```python
from build123d import *

# Parameters (mm, degrees)
SKETCH1_R           = 15
BOSS_EXTRUDE1_DEPTH = 40
BOSS_EXTRUDE2_START = 20
SKETCH2_R           = 20
BOSS_EXTRUDE2_DEPTH = 30
SKETCH3_R           = 15
BOSS_EXTRUDE3_DEPTH = 40


with BuildPart() as part:
    # Sketch1 → Boss-Extrude1 (new body)
    with BuildSketch(Plane(origin=(0, 0, 0), x_dir=(1, 0, 0), z_dir=(0, 1, 0))):
        with BuildLine():
            Line((-20, -20), (20, -20))
            Line((20, -20), (20, 0))
            ThreePointArc((20, 0), (0, 20), (-20, 0))
            Line((-20, 0), (-20, -20))
        make_face()
        with Locations(Location((0, 0, 0), (0, 0, 270))):
            Circle(SKETCH1_R, mode=Mode.SUBTRACT)
    extrude(amount=BOSS_EXTRUDE1_DEPTH)

    # Sketch2 → Boss-Extrude2 (add)
    with BuildSketch(Plane.XY.offset(BOSS_EXTRUDE2_START)):
        with Locations((0, 20)):
            Circle(SKETCH2_R)
    extrude(amount=BOSS_EXTRUDE2_DEPTH)

    # Sketch3 → Boss-Extrude3 (add)
    with BuildSketch(Plane.ZY.offset(20)):
        with BuildLine():
            Line((50, 40.055924185), (50, 0.055924185))
            Line((50, 0.055924185), (70, 0.055924185))
            ThreePointArc((70, 0.055924185), (90, 20.055924185), (70, 40.055924185))
            Line((70, 40.055924185), (50, 40.055924185))
        make_face()
        with Locations(Location((70, 20.055924185, 0), (0, 0, 270))):
            Circle(SKETCH3_R, mode=Mode.SUBTRACT)
    extrude(amount=-BOSS_EXTRUDE3_DEPTH)


solid = part.part
```
The listing builds one solid part. Answer for the finished solid, in the listing's coordinates (mm). A direction names the side the tool comes from. Round coordinates to 2 decimals unless told otherwise and drop trailing zeros. Order: outer loops, then holes, each group sorted by start corner. A loop starts at its lowest first (then second) coordinate and runs counter-clockwise, first axis right, second up. Notation, with made-up numbers: (-36, -4.5) -> (-21, -4.5) arc R20 cw to (-21, 20.5) -> close; hole circle Ø1 at (-13.5, 41.5). An arc over 180 degrees is marked (long way). Answer as CSV lines item,"result".
Q1. For a pull along Z with two mould halves and no side action, classify faces 1 (the flat face through (20, 20, 10)), 2 (the cylindrical face through (0, 20, -20)), 3 (the flat face through (-16, 35, 20)), 4 (the cylindrical face through (0, 20, 90)) as +Z half, -Z half, draft (parallel to the pull), parting line (faces both ways), or undercut.
Computed values:
face 1,"draft"
face 2,"-Z half"
face 3,"undercut"
face 4,"+Z half"
Q2. A cutting plane is placed at B-B on x = -13. Determine the outline of the cut face in (y, z).
Computed values:
outline,"(0, -15.2) -> (40, -15.2) -> (40, -7.48) -> (0, -7.48) -> close; (0, 7.48) -> (40, 7.48) -> (40, 20) -> (35.2, 20) -> (35.2, 50) -> (40.06, 50) -> (40.06, 70) arc R20 ccw to (0.06, 70) -> (0.06, 50) -> (4.8, 50) -> (4.8, 20) -> (0, 20) -> close; hole circle Ø30 at (20.06, 70)"
Q3. A cutting plane is placed at C-C on z = 63.5. Determine the outline of the cut face in (x, y).
Computed values:
outline,"(-20, 0.06) -> (20, 0.06) -> (20, 6.54) -> (-20, 6.54) -> close; (-20, 33.57) -> (20, 33.57) -> (20, 40.06) -> (-20, 40.06) -> close"
Q4. Given pin 1 (16 mm diameter, centred on x = 11.5, y = 33, fed in from +Z); pin 2 (1.5 mm diameter, centred on x = -4.5, z = 54, fed in from -Y); pin 3 (10 mm diameter, centred on x = 13.5, z = 3.5, fed in from +Y); pin 4 (18 mm diameter, centred on x = 0, z = 0, fed in from +Y), each flat-ended and moving along its own axis, determine where each tip first touches the part or whether it passes through.
Computed values:
pin 1,"stops at z = 89.38"
pin 2,"stops at y = 0.06"
pin 3,"stops at y = 40"
pin 4,"passes through"
Q5. A cutting plane is placed at D-D on y = 3.5. Determine the outline of the cut face in (x, z).
Computed values:
outline,"(-20, 0) arc R20 ccw to (20, 0) -> (20, 20) -> (11.3, 20) -> (11.3, 50) -> (20, 50) -> (20, 81.22) -> (-20, 81.22) -> (-20, 50) -> (-11.3, 50) -> (-11.3, 20) -> (-20, 20) -> close; hole circle Ø30 at (0, 0)"
Q6. Which of the six approach directions +Z, -Z, +X, -X, +Y, -Y give full straight-line access (tool end or side, diameter ignored) to faces 5 (the flat face through (4.4, 39.7, 50)), 6 (the flat face through (16, 4, 50)), 7 (the flat face through (16, 36, 20))?
Computed values:
face 5,"+Y"
face 6,"+X, -Y"
face 7,"+X, +Y"
Q7. A cutting plane is placed at A-A on y = 25.5. Determine the outline of the cut face in (x, z), plus the area to 3 significant figures.
Computed values:
outline,"(-20, 0) arc R20 ccw to (20, 0) -> (20, 20) -> (19.23, 20) -> (19.23, 50) -> (20, 50) -> (20, 56.02) -> (-20, 56.02) -> (-20, 50) -> (-19.23, 50) -> (-19.23, 20) -> (-20, 20) -> close; (-20, 83.98) -> (20, 83.98) -> (20, 89.24) -> (-20, 89.24) -> close; hole circle Ø30 at (0, 0)"
area,"2,330 mm^2"
Q8. Consider line 1 (X direction, y = 18, z = 0); line 2 (Z direction, x = -7, y = 22.5) (1 decimal); line 3 (Z direction, x = 7.5, y = 29.5). Determine where each line is inside the solid, lowest interval first. Write a range as from..to.
Computed values:
line 1,"x = -20..-15, 15..20"
line 2,"z = -18.7..-13.3, 13.3..55.2, 84.8..89.9"
line 3,"z = -18.54..-12.99, 12.99..58.35, 81.65..87.63"
